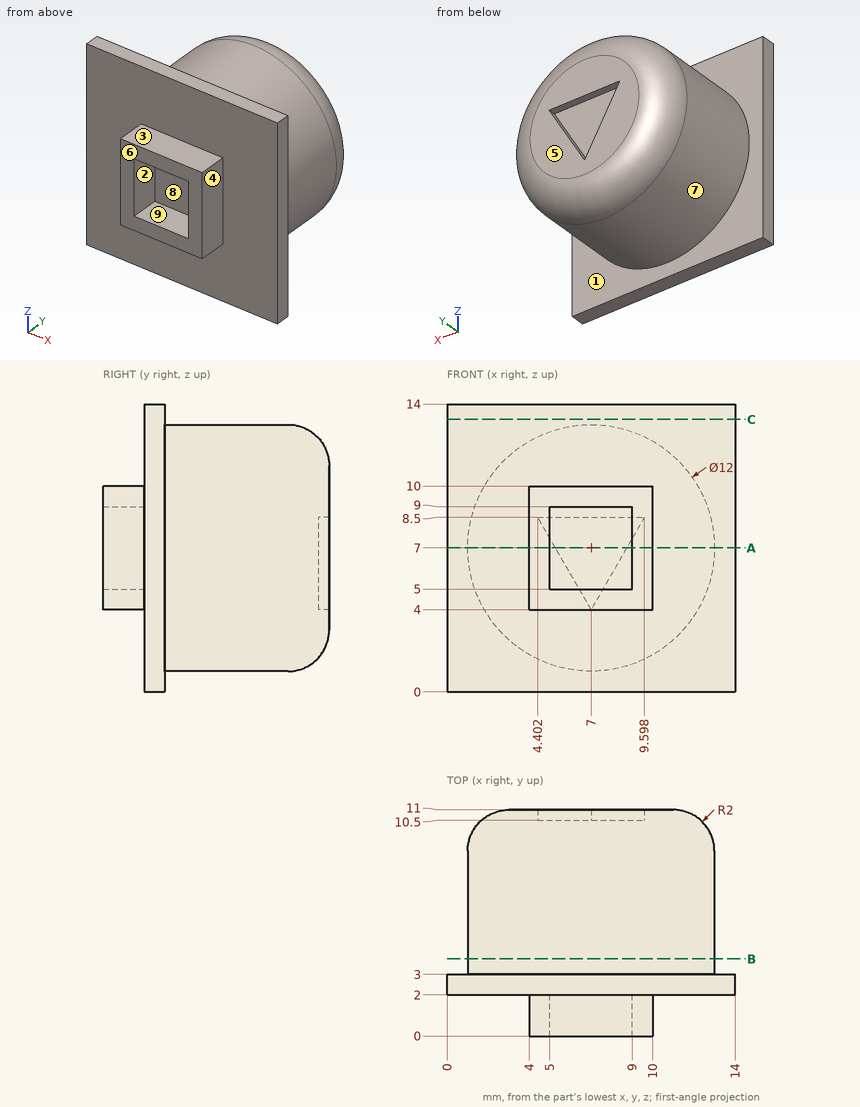
The drawing under review shows one solid part. Ordinate dimensions are in mm from its lowest x, y, z. A direction names the side the tool comes from. Give positions to 0.01 mm unless a question says otherwise; leave off trailing zeros. Write each loop counter-clockwise with the first axis right and the second up, starting at its lowest first coordinate (ties: lowest second). Pieces come first, ordered by that corner, then holes.
1. Add section B-B, the plane y = 3.75. Write out the cut boundary in (x, z), plus the area to 3 significant figures.
2. Tool access review of the marked faces 1, 2, 3, 4 and 5: name each direction out of +Z, -Z, +X, -X, +Y, -Y from which nothing blocks a thin tool from reaching the whole face with its end or side.
3. Wall thickness on L1, parallel to X at y = 1.5, z = 8.5; L2, parallel to Y at x = 7.25, z = 7; L3, parallel to Y at x = 12.75, z = 12: over which ranges is each line inside the solid? List them lowest first.
4. Add section C-C, the plane z = 13.25. Write out the cut boundary in (x, y), plus the area to 3 significant figures.
5. Draft analysis for pull direction X (two halves, no side actions). For the marked faces 6, 7, 8 and 9, state which applies: +X half, -X half, draft (parallel to the pull), parting line (faces both ways), or undercut.
6. For P1, Ø0.6, axis at y = 1, z = 8, coming from the +X side; P2, Ø4, axis at x = 7, z = 3, coming from the -Y side; P3, Ø1.6, axis at x = 7.5, y = 1, coming from the -Z side; P4, Ø1, axis at x = 6.5, y = 1, coming from the +Z side, all flat-tipped, find the tip position at first contact; note any pin that passes through.
7. Add section A-A, the plane z = 7. Write out the cut boundary in (x, y), plus the area to 3 significant figures.
Worked answers:
1. outline: circle Ø12 at (7, 7)
1. area: 113 mm2
2. face 1: +Y
2. face 2: -Y
2. face 3: +Z, +X, -X, -Y
2. face 4: +Z, -Z, +X, -Y
2. face 5: +Z, -Z, +X, -X, +Y
3. L1: x = 4 to 5, 9 to 10
3. L2: y = 2 to 10.5
3. L3: y = 2 to 3
4. outline: (0, 2) - (14, 2) - (14, 3) - (0, 3) - close
4. area: 14.0 mm2
5. face 6: draft
5. face 7: parting line
5. face 8: undercut
5. face 9: undercut
6. P1: stops at x = 10
6. P2: stops at y = 0
6. P3: stops at z = 4
6. P4: stops at z = 10
7. outline: (0, 2) - (4, 2) - (4, 0) - (5, 0) - (5, 2) - (9, 2) - (9, 0) - (10, 0) - (10, 2) - (14, 2) - (14, 3) - (13, 3) - (13, 9) arc R2 ccw to (11, 11) - (8.73, 11) - (8.73, 10.5) - (5.27, 10.5) - (5.27, 11) - (3, 11) arc R2 ccw to (1, 9) - (1, 3) - (0, 3) - close
7. area: 111 mm2
